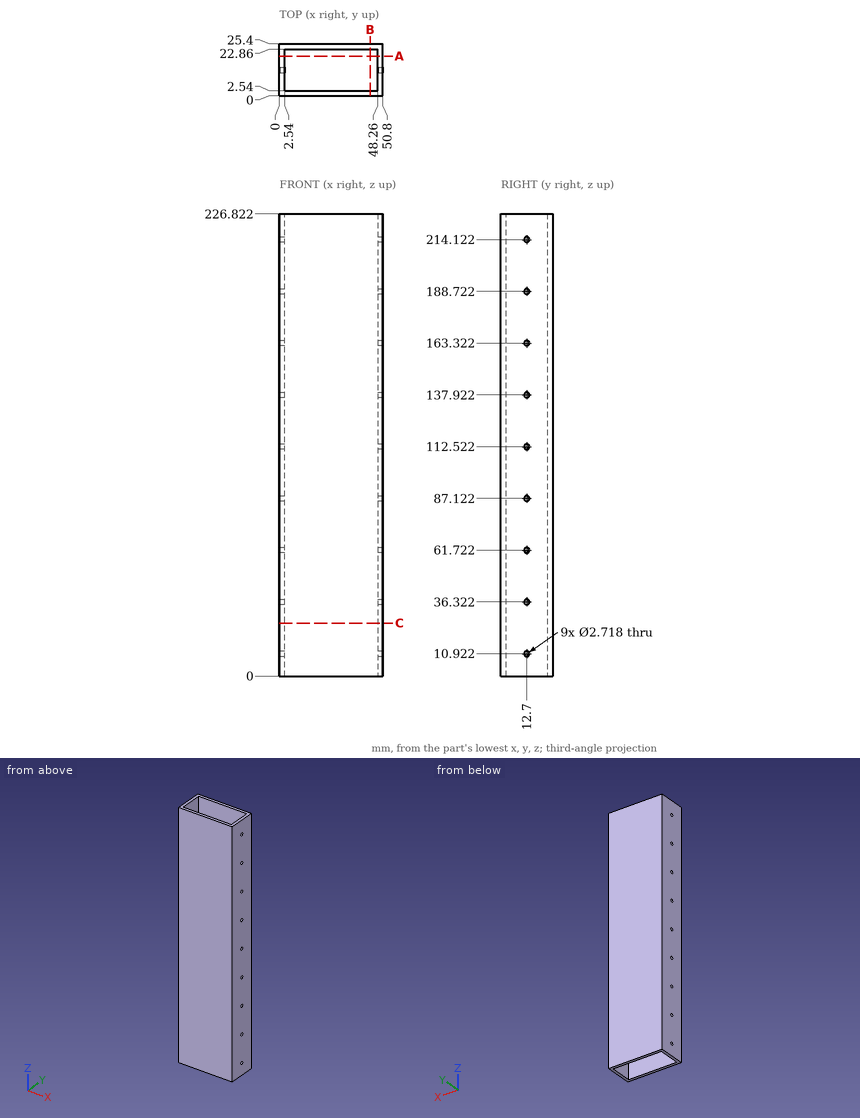
Part print with two shaded views. Sizes in mm from the minimum x, y, z corner. Coordinates: 2 decimals unless noted, no trailing zeros. Write each loop counter-clockwise with the first axis right and the second up, starting at its lowest first coordinate (ties: lowest second). Pieces come first, ordered by that corner, then holes.
1. Band-saw the part on B-B, the plane x = 44.5. Give the cut face in (y, z), and give its area (3 significant figures).
Answer block:
outline: (0, 0) - (2.54, 0) - (2.54, 226.82) - (0, 226.82) - close; (22.86, 0) - (25.4, 0) - (25.4, 226.82) - (22.86, 226.82) - close
area: 1,150 mm2
2. Drill centre lines: probe 1 along Y at (x, z) = (47.5, 90.5); probe 2 along X at (y, z) = (8.5, 144). Where is each one in solid material? Low to high.
Answer block:
probe 1: y = 0 to 2.54, 22.86 to 25.4
probe 2: x = 0 to 2.54, 48.26 to 50.8
3. Band-saw the part on A-A, the plane y = 19.5. Give the cut face in (x, z), and give its area (3 significant figures).
Answer block:
outline: (0, 0) - (2.54, 0) - (2.54, 226.82) - (0, 226.82) - close; (48.26, 0) - (50.8, 0) - (50.8, 226.82) - (48.26, 226.82) - close
area: 1,150 mm2
4. Band-saw the part on C-C, the plane z = 26. Give the cut face in (x, y), and give its area (3 significant figures).
Answer block:
outline: (0, 0) - (50.8, 0) - (50.8, 25.4) - (0, 25.4) - close; hole (2.54, 2.54) - (48.26, 2.54) - (48.26, 22.86) - (2.54, 22.86) - close
area: 361 mm2
5. Drop a flat-ended pin along its axis: pin 1 (2 mm diameter, centred on x = 21.5, y = 22.5, fed in from -Z). Give the stop position or say it passes through.
Answer block:
pin 1: stops at z = 0
